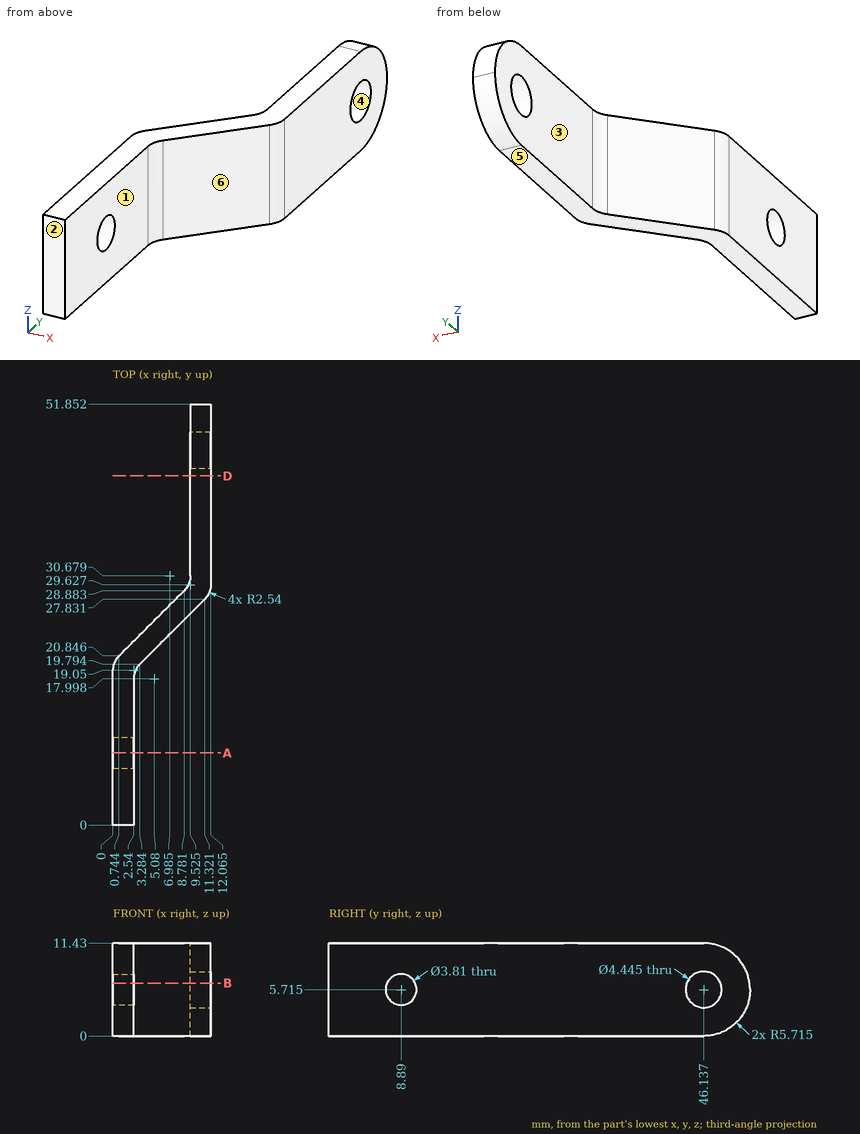
Input: dimensioned drawing with shaded views. Units: mm. Origin: part minimum x, y, z. A direction names the side the tool comes from. Round coordinates to 2 decimals unless told otherwise and drop trailing zeros. Order: outer loops, then holes, each group sorted by start corner. A loop starts at its lowest first (then second) coordinate and runs counter-clockwise, first axis right, second up. Notation, with made-up numbers: (37.25, 67.25) - (42.25, 67.25) arc R15 cw to (42.25, 86.25) - close; hole circle Ø11 at (68, 88). An arc over 180 degrees is marked (long way). Write item = value, one per line. Start each with the question number.
Q1. Cut plane B-B on z = 6.5. Give the number of separate pieces and of enclosed holes in the cut face, and give its area (3 significant figures).
Q2. Pin query (flat end, axial travel): pin 1 (4 mm diameter, centred on y = 45, z = 5.5, fed in from -X) (3 decimals); pin 2 (3.5 mm diameter, centred on y = 6, z = 7, fed in from +X); pin 3 (1 mm diameter, centred on x = 2.5, z = 8, fed in from -Y); pin 4 (1.5 mm diameter, centred on y = 17.5, z = 9, fed in from +X). Return the tip coordinate at first contact, or that it passes through.
Q3. Cut plane A-A on y = 8.89. Return the cut outline in (x, z).
Q4. Access query for the marked faces 1, 2 and 3. Directions: +Z, -Z, +X, -X, +Y, -Y. A direction counts if a zero-diameter tool reaches every point of the face in a straight line with its end or side. Return the directions, or none.
Q5. Pull-direction query (Y, two-part tool) for the marked faces 4, 5 and 6; classes: +Y half, -Y half, draft (parallel to the pull), parting line (faces both ways), or undercut.
Q6. Cut plane D-D on y = 43. Return the cut outline in (x, z) (3 decimals).
Q7. Ray query, line 1 (X direction, y = 17, z = 4); line 2 (X direction, y = 31, z = 2.5) (3 decimals); line 3 (Z direction, x = 2, y = 7.5). Return the intervals inside material, ascending. Write a range as from..to.
Outcome:
q1.separate_pieces = 3
q1.enclosed_holes = 0
q1.area = 122 mm^2
q2.pin_1 = 9.525
q2.pin_2 = 2.54
q2.pin_3 = 0
q2.pin_4 = 2.55
q3.outline = (0, 0) - (2.54, 0) - (2.54, 3.81) - (0, 3.81) - close; (0, 7.62) - (2.54, 7.62) - (2.54, 11.43) - (0, 11.43) - close
q4.face_1 = +Z, -Z, +X, -Y
q4.face_2 = +Z, -Z, +X, -X, -Y
q4.face_3 = +Z, -Z, -X, +Y
q5.face_4 = undercut
q5.face_5 = draft
q5.face_6 = -Y half
q6.outline = (9.525, 0) - (12.065, 0) - (12.065, 11.43) - (9.525, 11.43) - close
q7.line_1 = 0..2.54
q7.line_2 = 9.525..12.065
q7.line_3 = 0..4.41, 7.02..11.43
